Could you check a few things on this model? Use its own coordinates, in mm. A direction names the side the tool comes from. Round coordinates to 2 decimals unless told otherwise and drop trailing zeros. Loops run counter-clockwise (first coordinate to the right, second up) from the corner with the lowest first, then second, coordinate; pieces in that order, holes last. Notation, with made-up numbers: M 71.25,-36.75 L 102.25,-36.75 A21 cw 102.25,-6.75 Z; hole C 28.5,75 d10. An arc over 180 degrees is marked long. One line per item, written item: value. Start each with the question number.
Q1. Please list where these lines run through material, in increasing order: line 1 along Y through (x, z) = (-2.5, 0.75); line 2 along X through (y, z) = (-12, 2); line 3 along X through (y, z) = (-16.5, 5.75).
Q2. I'm going to push flat-ended pins straight in: pin 1 Ø3.5 at (x, z) = (-17, 6.5) entering from -Y; pin 2 Ø0.6 at (y, z) = (2, 7.5) entering from +X; pin 3 Ø1.2 at (x, z) = (16, 5.5) entering from +Y. Where does each tip first touch, or does it pass through?
Q3. Thinking about a two-plate mould opening in Y: for faces 1 (the face through (-24, 5, 3)), 2 (the face through (-17, 3.5, 5)), 3 (the face through (5, 21.5, 2)), which applies, released by +Y, released by -Y, zero draft, split by the parting line, or undercut?
Q4. Imagine slicing it at B-B (y = 1). Please give me the cut outline in (x, z), then the cut area to 3 significant figures.
Q5. Which directions (+Z, -Z, +X, -X, +Y, -Y) give clear straight access to the entire face, cutting with the end or side of a thin tool? Please do faces 4 (the face through (-17, -3.5, 5)), 5 (the face through (5, -21, 4.5)), 6 (the face through (-17, 5, 8)), 7 (the face through (-19.5, 17, 3)), 8 (the face through (-20, -4, 8)).
Q6. Imagine slicing it at A-A (z = 3.75). Please give me the cut outline in (x, y).
Q7. Imagine slicing it at D-D (z = 8). Please give me the cut outline in (x, y).
Q8. Imagine slicing it at C-C (x = 17.75). Please give me the cut outline in (y, z), then the cut area to 3 significant figures.
from build123d import *

# Parameters (mm, degrees)
F1_DEPTH = 7
F2_W     = 39
F2_H     = 1
F3_DEPTH = 50
F5_DEPTH = 2
F6_W     = 1.5
F6_H     = 2.5
F7_DEPTH = 50


with BuildPart() as f1:
    # F0 (on Top) → F1 (new body)
    with BuildSketch(Plane.XY):
        Polygon((-19.5, -21.5), (28.5, -21.5), (28.5, 21.5), (-19.5, 21.5), (-19.5, 12.5), (-24, 8), (-24, 2), (-18.5, 2), (-18.5, 3.5), (-15.5, 3.5), (-15.5, 2), (-15.5, 0), (-15.5, -2), (-15.5, -3.5), (-18.5, -3.5), (-18.5, -2), (-24, -2), (-24, -8), (-19.5, -12.5), align=None)
        with BuildLine():
            Line((20, 5), (20, -14))
            Line((20, -14), (20, -16.25))
            ThreePointArc((20, -16.25), (17.75, -18.5), (15.5, -16.25))
            Line((15.5, -16.25), (15.5, -14))
            Line((15.5, -14), (15.5, 5))
            ThreePointArc((15.5, 5), (14.823785, 10.240299), (12.839445, 15.137277))
            ThreePointArc((12.839445, 15.137277), (13.105805, 18.044603), (16.010887, 17.754792))
            ThreePointArc((16.010887, 17.754792), (17.529097, 15.504906), (18.639882, 13.028395))
            ThreePointArc((18.639882, 13.028395), (19.657565, 9.071396), (20, 5))
        make_face(mode=Mode.SUBTRACT)
    extrude(amount=F1_DEPTH)

    # F2 (on face) → F3 (cut)
    with BuildSketch(Plane.YZ.offset(28.5)):
        with Locations((0, 0.5)):
            Rectangle(F2_W, F2_H)
    extrude(amount=-F3_DEPTH, mode=Mode.SUBTRACT)

    # F4 (on face) → F5 (join)
    with BuildSketch(Plane.XY.offset(7)):
        Polygon((-24, -2), (-24, -3.5), (-20, -3.5), (-20, -5), (-14, -5), (-14, 5), (-20, 5), (-20, 3.5), (-24, 3.5), (-24, 2), (-18.5, 2), (-18.5, 3.5), (-15.5, 3.5), (-15.5, -3.5), (-18.5, -3.5), (-18.5, -2), align=None)
    extrude(amount=F5_DEPTH)

    # F6 (on face) → F7 (cut)
    with BuildSketch(Plane.YZ.offset(28.5)):
        with Locations((-20.75, 5.75)):
            Rectangle(F6_W, F6_H)
        with Locations((20.75, 5.75)):
            Rectangle(F6_W, F6_H)
    extrude(amount=-F7_DEPTH, mode=Mode.SUBTRACT)


solid = f1.part
Report:
1. line 1: y = -21.5 to -19.5, 19.5 to 21.5
1. line 2: x = -20 to 15.5, 20 to 28.5
1. line 3: x = -19.5 to 15.51, 19.99 to 28.5
2. pin 1: stops at y = -20
2. pin 2: stops at x = -14
2. pin 3: stops at y = 20
3. face 1: zero draft
3. face 2: undercut
3. face 3: released by +Y
4. outline: M -15.5,1 L 15.5,1 L 15.5,7 L -14,7 L -14,9 L -15.5,9 Z; M 20,1 L 28.5,1 L 28.5,7 L 20,7 Z
4. area: 240 mm²
5. face 4: +Z, -Z
5. face 5: +Z, +X, -X, -Y
5. face 6: +Z, +X, -X, +Y
5. face 7: +Z, -Z, -X, +Y
5. face 8: +Z, -X, -Y
6. outline: M -24,-8 L -19.5,-12.5 L -19.5,-21.5 L 28.5,-21.5 L 28.5,21.5 L -19.5,21.5 L -19.5,12.5 L -24,8 L -24,2 L -18.5,2 L -18.5,3.5 L -15.5,3.5 L -15.5,-3.5 L -18.5,-3.5 L -18.5,-2 L -24,-2 Z; hole M 12.84,15.14 A20.64 cw 15.5,5 L 15.5,-16.25 A2.25 ccw 20,-16.25 L 20,5 A24.37 ccw 18.64,13.03 A15.8 ccw 16.01,17.75 A2.06 ccw long Z
7. outline: M -24,-3.5 L -20,-3.5 L -20,-5 L -14,-5 L -14,5 L -20,5 L -20,3.5 L -24,3.5 L -24,2 L -18.5,2 L -18.5,3.5 L -15.5,3.5 L -15.5,-3.5 L -18.5,-3.5 L -18.5,-2 L -24,-2 Z
8. outline: M -21.5,0 L -19.5,0 L -19.5,1 L -18.5,1 L -18.5,7 L -20,7 L -20,4.5 L -21.5,4.5 Z; M 15.09,1 L 19.5,1 L 19.5,0 L 21.5,0 L 21.5,4.5 L 20,4.5 L 20,7 L 15.09,7 Z
8. area: 52.9 mm²
